from build123d import *

# Parameters (mm, degrees)
CROQUIS4_R              = 10.9
SALIENTE_EXTRUIR3_DEPTH = 1.35


with BuildPart() as part:
    # Croquis1 → Revolución1 (revolve)
    with BuildSketch(Plane.XY):
        Polygon((-10.9, 20), (-10.9, 0), (-12.25, 0), (-12.25, 18), (-22.25, 18), (-12.25, 20), align=None)
    revolve(axis=Axis((0, 0, 0), (0, 1, 0)))

    # Croquis4 → Saliente-Extruir3 (add)
    with BuildSketch(Plane(origin=(0, 20, 0), x_dir=(1, 0, 0), z_dir=(0, 1, 0))):
        Circle(CROQUIS4_R)
    extrude(amount=-SALIENTE_EXTRUIR3_DEPTH)


solid = part.part
Geometry check sheet. Reference: the model listing, model coordinates, mm. A direction names the side the tool comes from. Coordinates: 2 decimals unless noted, no trailing zeros. Order: outer loops, then holes, each group sorted by start corner. A loop starts at its lowest first (then second) coordinate and runs counter-clockwise, first axis right, second up. Notation, with made-up numbers: (8, 59.5) -> (24, 59.5) arc R23 cw to (24, 84.5) -> close; hole circle Ø9 at (-3, 28). An arc over 180 degrees is marked (long way). Use a Markdown table: item, result. Add a question column.
1. Cross-section at B-B (y = 12.5). Enter the section's corners in (x, z).
2. Go/stop test with flat-tipped pins: pin 1 Ø10 at (x, y) = (-17.5, 12.5) entering from +Z; pin 2 Ø10 at (x, y) = (10.5, 4) entering from -Z; pin 3 Ø11 at (x, z) = (-3.5, -0.5) entering from -Y; pin 4 Ø2 at (y, z) = (15, 8) entering from -X. Record where each tip stops, or that it passes through.
3. Mould release check, pull along Z, two halves, no side actions. Record for faces 3 (the face through (-10.4, 9.19, 3.27)), 4 (the face through (-6.586, 9.126, 10.329)), 5 (the face through (0, 20, 0)): pulls with the +Z half, pulls with the -Z half, needs draft (parallel to the pull), parting line crosses it, or undercut.
4. Material ranges on L1, parallel to Z at x = 0, y = 13.25; L2, parallel to Y at x = -10, z = 0; L3, parallel to Z at x = 9.5, y = 2.5, recorded low to high.
5. Set-up check for faces 1 (the face through (-11, 0, -2)), 2 (the face through (10, 18, -10)): record each of +Z, -Z, +X, -X, +Y, -Y from which the full face is reachable in a straight line by a thin tool's end or side.
6. Cross-section at A-A (x = 0). Enter the section's corners in (y, z).
Filled sheet:
| question | item | result |
|---|---|---|
| 1 | outline | circle Ø24.5 at (0, 0); hole circle Ø21.8 at (0, 0) |
| 2 | pin 1 | through |
| 2 | pin 2 | z = -10.95 |
| 2 | pin 3 | y = 18.65 |
| 2 | pin 4 | x = -10.05 |
| 3 | face 3 | undercut |
| 3 | face 4 | parting line crosses it |
| 3 | face 5 | needs draft |
| 4 | L1 | -12.25 to -10.9, 10.9 to 12.25 |
| 4 | L2 | 18.65 to 20 |
| 4 | L3 | -7.73 to -5.34, 5.34 to 7.73 |
| 5 | face 1 | +Z, -Z, +X, -X, -Y |
| 5 | face 2 | -Y |
| 6 | outline | (0, -12.25) -> (18, -12.25) -> (18, -22.25) -> (20, -12.25) -> (20, 12.25) -> (18, 22.25) -> (18, 12.25) -> (0, 12.25) -> (0, 10.9) -> (18.65, 10.9) -> (18.65, -10.9) -> (0, -10.9) -> close |
